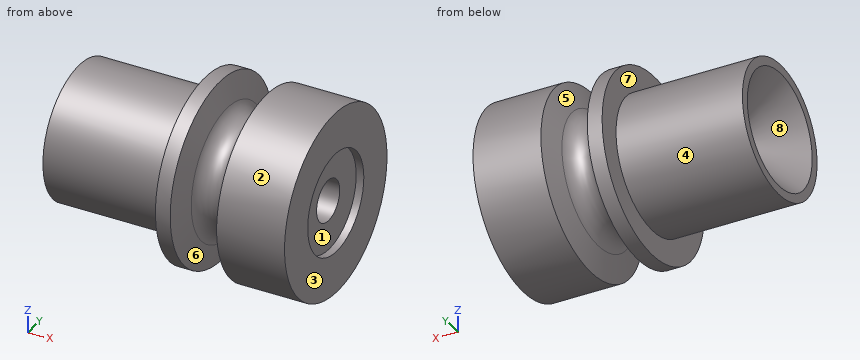
from build123d import *


with BuildPart() as part:
    # Sketch1 → Revolve1 (revolve)
    with BuildSketch(Plane.XY):
        with BuildLine():
            Line((-7.83533025, 7.706480957), (-7.041793614, 10.668))
            Line((-7.041793614, 10.668), (0.892, 10.668))
            Line((0.892, 10.668), (0.892, 5.842))
            Line((0.892, 5.842), (0, 5.842))
            Line((0, 5.842), (0, 2.413))
            Line((0, 2.413), (-24.6126, 2.413))
            Line((-24.6126, 2.413), (-28.956, 6.7564))
            Line((-28.956, 6.7564), (-28.956, 7.7724))
            Line((-28.956, 7.7724), (-14.188119198, 7.7724))
            Line((-14.188119198, 7.7724), (-14.188119198, 10.668))
            Line((-14.188119198, 10.668), (-12.462385009, 10.668))
            Line((-12.462385009, 10.668), (-11.668848373, 7.706480957))
            ThreePointArc((-11.668848373, 7.706480957), (-9.752089311, 6.2357), (-7.83533025, 7.706480957))
        make_face()
    revolve(axis=Axis((-22.598839253, 0, 0), (1, 0, 0)))


solid = part.part
Can you work these out from the model? Positions are in its coordinate system, mm. Face numbers are marked on the shaded views. A direction names the side the tool comes from. Round coordinates to 2 decimals unless told otherwise and drop trailing zeros. Write each loop counter-clockwise with the first axis right and the second up, starting at its lowest first coordinate (ties: lowest second). Pieces come first, ordered by that corner, then holes. Notation, with made-up numbers: (22, -3) -> (54, -3) arc R30 ccw to (54, 23) -> close; hole circle Ø8 at (47.5, 80.25). An arc over 180 degrees is marked (long way). One line per question, with ' | ' between items. Start each with the question number.
1) I'm going to push flat-ended pins straight in: P1, Ø6, axis at x = -25.5, y = 7.5, coming from the -Z side; P2, Ø6, axis at y = -1.5, z = -1.5, coming from the +X side; P3, Ø1.5, axis at x = -15.5, z = -4.5, coming from the +Y side; P4, Ø4, axis at y = 0, z = 0, coming from the +X side. Where does each tip first touch, or does it pass through?
2) On a 3-axis mill with a long thin cutter (end or side, diameter ignored), from which of +Z, -Z, +X, -X, +Y, -Y can I reach the whole of each face in a straight line? I mean the marked faces 1, 2, 3, 4 and 5. Say none if no direction works.
3) Suppose I cut it at C-C on x = -17.75. Write out the boundary of the cut face in (y, z), then the cut area to 3 significant figures.
4) Suppose I cut it at A-A on z = 0. Write out the boundary of the cut face in (x, y).
5) Suppose I cut it at D-D on x = -1.25. Write out the boundary of the cut face in (y, z).
6) I need wall thicknesses on line 1 (Z direction, x = 0.5, y = 0); line 2 (X direction, y = 4.5, z = -5.5); line 3 (X direction, y = -2.25, z = -7.5). Which ranges of each line are inside material? Lowest first, please. Write a range as [from, to].
7) If we mould it in two halves opening along Z, with no side actions, what happens to the marked faces 6, 7 and 8? For each: released by +Z, released by -Z, zero draft, split by the parting line, or undercut.
Return value:
1) P1: stops at z = -6.34 | P2: stops at x = 0 | P3: stops at y = 6.81 | P4: passes through
2) face 1: +X | face 2: +X, -X | face 3: +Z, -Z, +X, +Y, -Y | face 4: -X | face 5: none
3) outline: circle Ø15.54 at (0, 0); hole circle Ø4.83 at (0, 0) | area: 171 mm2
4) outline: (-28.96, -7.77) -> (-14.19, -7.77) -> (-14.19, -10.67) -> (-12.46, -10.67) -> (-11.67, -7.71) arc R1.98 cw to (-7.84, -7.71) -> (-7.04, -10.67) -> (0.89, -10.67) -> (0.89, -5.84) -> (0, -5.84) -> (0, -2.41) -> (-24.61, -2.41) -> (-28.96, -6.76) -> close; (-28.96, 6.76) -> (-24.61, 2.41) -> (0, 2.41) -> (0, 5.84) -> (0.89, 5.84) -> (0.89, 10.67) -> (-7.04, 10.67) -> (-7.84, 7.71) arc R1.98 cw to (-11.67, 7.71) -> (-12.46, 10.67) -> (-14.19, 10.67) -> (-14.19, 7.77) -> (-28.96, 7.77) -> close
5) outline: circle Ø21.34 at (0, 0); hole circle Ø4.83 at (0, 0)
6) line 1: z = [-10.67, -5.84], [5.84, 10.67] | line 2: x = [-28.96, -11.39], [-8.11, 0.89] | line 3: x = [-14.19, -11.7], [-7.8, 0.89]
7) face 6: split by the parting line | face 7: zero draft | face 8: undercut
